from build123d import *

# Parameters (mm, degrees)
SKETCH021_W     = 65
SKETCH021_H     = 85
PAD015_DEPTH    = 63
SKETCH022_W     = 40
SKETCH022_H     = 85
POCKET009_DEPTH = 53.7
SKETCH023_W     = 37.5
SKETCH023_H     = 60
POCKET010_DEPTH = 63


with BuildPart() as part:
    # Sketch021 → Pad015 (new body)
    with BuildSketch(Plane.XY):
        with Locations((0, -30)):
            Rectangle(SKETCH021_W, SKETCH021_H)
    extrude(amount=PAD015_DEPTH)

    # Sketch022 (on Face5 of Pad015) → Pocket009 (cut)
    with BuildSketch(Plane(origin=(0, 0, 0), x_dir=(1, 0, 0), z_dir=(0, 0, -1))):
        with Locations((0, 30)):
            Rectangle(SKETCH022_W, SKETCH022_H)
    extrude(amount=-POCKET009_DEPTH, mode=Mode.SUBTRACT)

    # Sketch023 → Pocket010 (cut)
    with BuildSketch(Plane.XY):
        with Locations((0, -30)):
            Rectangle(SKETCH023_W, SKETCH023_H)
    extrude(amount=POCKET010_DEPTH, mode=Mode.SUBTRACT)


with BuildPart() as part_1:
    # Body003 placement: moved
    add(part.part.moved(Location((0, 0, 15))))


solid = part_1.part
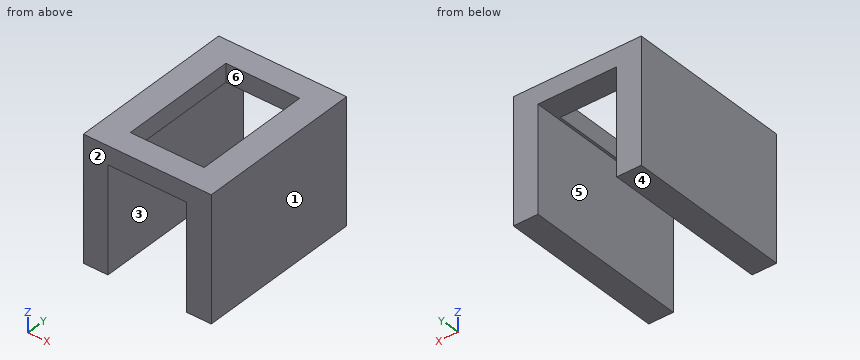
CAD build for the part. Positions are in the model's coordinates, mm. Face numbers are marked on the shaded views. A direction names the side the tool comes from. Coordinates: 2 decimals unless noted, no trailing zeros. Write each loop counter-clockwise with the first axis right and the second up, starting at its lowest first coordinate (ties: lowest second). Pieces come first, ordered by that corner, then holes. Notation, with made-up numbers: M 30,67.25 L 40,67.25 A25 cw 40,99.25 Z; hole C -13.5,-22 d1. An arc over 180 degrees is marked long. Return JSON: item names as keys, results as strings.
Item 1: Slice it at A-A, the plane z = 58.5. Write the cut outline in (x, y).
Findings below:
{"outline": "M -32.5,-72.5 L -20,-72.5 L -20,12.5 L -32.5,12.5 Z; M 20,-72.5 L 32.5,-72.5 L 32.5,12.5 L 20,12.5 Z"}
Item 2: Drop flat-ended pins along their axis: pin 1 Ø1.5 at (x, y) = (9, -61) entering from -Z; pin 2 Ø4 at (x, y) = (-16, -47) entering from +Z. Give the stop position or say it passes through.
Findings below:
{"pin 1": "stops at z = 68.7", "pin 2": "passes through"}
Item 3: Probe line 1 (X direction, y = -69, z = 49); line 2 (X direction, y = -11, z = 73); line 3 (Y direction, x = 10.5, z = 73). List the from-to ranges inside material, lowest first. Write a range as from..to.
Findings below:
{"line 1": "x = -32.5..-20, 20..32.5", "line 2": "x = -32.5..-18.75, 18.75..32.5", "line 3": "y = -72.5..-60, 0..12.5"}
Item 4: Slice it at C-C, the plane x = -8.5. Write the cut outline in (y, z), and give its area (4 significant figures).
Findings below:
{"outline": "M -72.5,68.7 L -60,68.7 L -60,78 L -72.5,78 Z; M 0,68.7 L 12.5,68.7 L 12.5,78 L 0,78 Z", "area": "232.5 mm2"}
Item 5: Slice it at B-B, the plane y = -47.5. Write the cut outline in (x, z).
Findings below:
{"outline": "M -32.5,15 L -20,15 L -20,68.7 L -18.75,68.7 L -18.75,78 L -32.5,78 Z; M 18.75,68.7 L 20,68.7 L 20,15 L 32.5,15 L 32.5,78 L 18.75,78 Z"}
Item 6: Slice it at D-D, the plane y = -67. Write the cut outline in (x, z).
Findings below:
{"outline": "M -32.5,15 L -20,15 L -20,68.7 L 20,68.7 L 20,15 L 32.5,15 L 32.5,78 L -32.5,78 Z"}
Item 7: Two-plate mould, pull along X, no slides. Class the marked faces 1, 2 and 3: +X half, -X half, draft (parallel to the pull), parting line (faces both ways), or undercut.
Findings below:
{"face 1": "+X half", "face 2": "draft", "face 3": "undercut"}
Item 8: Which spindle directions (+Z, -Z, +X, -X, +Y, -Y) get a long thin tool onto all of the face, cutting with end or side? Do the marked faces 4, 5 and 6. Say none if no direction does.
Findings below:
{"face 4": "-Z, +X, -X, +Y, -Y", "face 5": "-Z, +Y, -Y", "face 6": "+Z, -Z"}
